```python
from build123d import *

# Parameters (mm, degrees)
BOSS_EXTRUDE1_DEPTH = 9
CUT_EXTRUDE1_DEPTH  = 1.6
CUT_EXTRUDE2_DEPTH  = 9
CUT_EXTRUDE4_DEPTH  = 6


with BuildPart() as part:
    # Sketch1 → Boss-Extrude1 (new body)
    with BuildSketch(Plane.XY):
        with BuildLine():
            Line((-290.5, 206.4), (290.5, 206.4))
            ThreePointArc((290.5, 206.4), (296.863961031, 203.763961031), (299.5, 197.4))
            Line((299.5, 197.4), (299.5, 0))
            ThreePointArc((299.5, 0), (296.863961031, -6.363961031), (290.5, -9))
            Line((290.5, -9), (-290.5, -9))
            ThreePointArc((-290.5, -9), (-296.863961031, -6.363961031), (-299.5, 0))
            Line((-299.5, 0), (-299.5, 197.4))
            ThreePointArc((-299.5, 197.4), (-296.863961031, 203.763961031), (-290.5, 206.4))
        make_face()
    extrude(amount=BOSS_EXTRUDE1_DEPTH)

    # Sketch4 → Cut-Extrude1 (cut)
    with BuildSketch(Plane.XY.offset(9)):
        with BuildLine():
            Line((-280.5, -4), (280.5, -4))
            ThreePointArc((280.5, -4), (290.399494937, 0.100505063), (294.5, 10))
            Line((294.5, 10), (294.5, 187.4))
            ThreePointArc((294.5, 187.4), (290.399494937, 197.299494937), (280.5, 201.4))
            Line((280.5, 201.4), (-280.5, 201.4))
            ThreePointArc((-280.5, 201.4), (-290.399494937, 197.299494937), (-294.5, 187.4))
            Line((-294.5, 187.4), (-294.5, 10))
            ThreePointArc((-294.5, 10), (-290.399494937, 0.100505063), (-280.5, -4))
        make_face()
        with BuildLine():
            Line((-280.5, 5), (280.5, 5))
            ThreePointArc((280.5, 5), (284.035533906, 6.464466094), (285.5, 10))
            Line((285.5, 10), (285.5, 187.4))
            ThreePointArc((285.5, 187.4), (284.035533906, 190.935533906), (280.5, 192.4))
            Line((280.5, 192.4), (-280.5, 192.4))
            ThreePointArc((-280.5, 192.4), (-284.035533906, 190.935533906), (-285.5, 187.4))
            Line((-285.5, 187.4), (-285.5, 10))
            ThreePointArc((-285.5, 10), (-284.035533906, 6.464466094), (-280.5, 5))
        make_face(mode=Mode.SUBTRACT)
    extrude(amount=-CUT_EXTRUDE1_DEPTH, mode=Mode.SUBTRACT)

    # Sketch5 → Cut-Extrude2 (cut)
    with BuildSketch(Plane.XY):
        with BuildLine():
            Line((-264.5, 177.4), (-26, 177.4))
            ThreePointArc((-26, 177.4), (-21.757359313, 175.642640687), (-20, 171.4))
            Line((-20, 171.4), (-20, 26))
            ThreePointArc((-20, 26), (-21.757359313, 21.757359313), (-26, 20))
            Line((-26, 20), (-264.5, 20))
            ThreePointArc((-264.5, 20), (-268.742640687, 21.757359313), (-270.5, 26))
            Line((-270.5, 26), (-270.5, 171.4))
            ThreePointArc((-270.5, 171.4), (-268.742640687, 175.642640687), (-264.5, 177.4))
        make_face()
        with BuildLine():
            Line((20, 171.4), (20, 26))
            ThreePointArc((20, 26), (21.757359313, 21.757359313), (26, 20))
            Line((26, 20), (163.5, 20))
            ThreePointArc((163.5, 20), (167.742640687, 21.757359313), (169.5, 26))
            Line((169.5, 26), (169.5, 171.4))
            ThreePointArc((169.5, 171.4), (167.742640687, 175.642640687), (163.5, 177.4))
            Line((163.5, 177.4), (26, 177.4))
            ThreePointArc((26, 177.4), (21.757359313, 175.642640687), (20, 171.4))
        make_face()
    extrude(amount=CUT_EXTRUDE2_DEPTH, mode=Mode.SUBTRACT)

    # Sketch7 → Cut-Extrude4 (cut)
    with BuildSketch(Plane(origin=(0, 0, 0), x_dir=(-1, 0, 0), z_dir=(0, 0, -1))):
        with BuildLine():
            Line((280.5, 26), (280.5, 171.4))
            ThreePointArc((280.5, 171.4), (275.813708499, 182.713708499), (264.5, 187.4))
            Line((264.5, 187.4), (26, 187.4))
            ThreePointArc((26, 187.4), (14.686291501, 182.713708499), (10, 171.4))
            Line((10, 171.4), (10, 26))
            ThreePointArc((10, 26), (14.686291501, 14.686291501), (26, 10))
            Line((26, 10), (264.5, 10))
            ThreePointArc((264.5, 10), (275.813708499, 14.686291501), (280.5, 26))
        make_face()
        with BuildLine():
            Line((-163.5, 10), (-26, 10))
            ThreePointArc((-26, 10), (-14.686291501, 14.686291501), (-10, 26))
            Line((-10, 26), (-10, 171.4))
            ThreePointArc((-10, 171.4), (-14.686291501, 182.713708499), (-26, 187.4))
            Line((-26, 187.4), (-163.5, 187.4))
            ThreePointArc((-163.5, 187.4), (-174.813708499, 182.713708499), (-179.5, 171.4))
            Line((-179.5, 171.4), (-179.5, 26))
            ThreePointArc((-179.5, 26), (-174.813708499, 14.686291501), (-163.5, 10))
        make_face()
    extrude(amount=-CUT_EXTRUDE4_DEPTH, mode=Mode.SUBTRACT)


solid = part.part
```
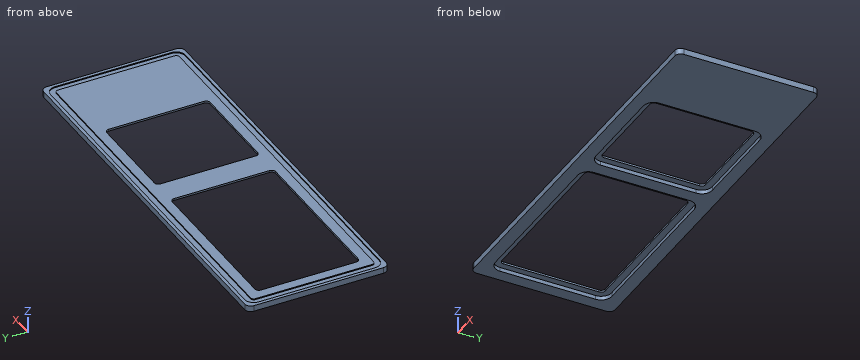
The listing builds one solid part. Answer for the finished solid, in the listing's coordinates (mm). Give positions to 0.01 mm unless a question says otherwise; leave off trailing zeros. Order: outer loops, then holes, each group sorted by start corner. A loop starts at its lowest first (then second) coordinate and runs counter-clockwise, first axis right, second up. Notation, with made-up numbers: (-14.5, 16.5) - (10.5, 16.5) arc R13 ccw to (10.5, 37.5) - close; hole circle Ø10 at (70, 42). An arc over 180 degrees is marked (long way). Answer in a Markdown table with one row per item. Add a question column.
Q1. The part is cut by section C-C (x = -210). Determine the outline of the cut face in (y, z), then the cut area to 3 significant figures.
Q2. Given P1, Ø1, axis at x = 184, y = 30.5, coming from the -Z side, flat-ended and moving along its own axis, determine where the tip first touches the part or whether it passes through.
Q3. The part is cut by section B-B (y = 133.5). Determine the outline of the cut face in (x, z), then the cut area to 3 significant figures.
Q4. Find the intervals of material crossed by line 1 along X through (y, z) = (142, 6.5); line 2 along Y through (x, z) = (77, 8); line 3 along X through (y, z) = (136, 4.5), in increasing order. Write a range as [from, to].
Q5. The part is cut by section A-A (z = 2). Determine the outline of the cut face in (x, y).
Determined:
| question | item | result |
|---|---|---|
| 1 | outline | (-9, 0) - (10, 0) - (10, 6) - (20, 6) - (20, 9) - (5, 9) - (5, 7.4) - (-4, 7.4) - (-4, 9) - (-9, 9) - close; (177.4, 6) - (187.4, 6) - (187.4, 0) - (206.4, 0) - (206.4, 9) - (201.4, 9) - (201.4, 7.4) - (192.4, 7.4) - (192.4, 9) - (177.4, 9) - close |
| 1 | area | 373 mm² |
| 2 | P1 | stops at z = 0 |
| 3 | outline | (-299.5, 0) - (-280.5, 0) - (-280.5, 6) - (-270.5, 6) - (-270.5, 9) - (-285.5, 9) - (-285.5, 7.4) - (-294.5, 7.4) - (-294.5, 9) - (-299.5, 9) - close; (-20, 6) - (-10, 6) - (-10, 0) - (10, 0) - (10, 6) - (20, 6) - (20, 9) - (-20, 9) - close; (169.5, 6) - (179.5, 6) - (179.5, 0) - (299.5, 0) - (299.5, 9) - (294.5, 9) - (294.5, 7.4) - (285.5, 7.4) - (285.5, 9) - (169.5, 9) - close |
| 3 | area | 1,520 mm² |
| 4 | line 1 | x = [-299.5, -270.5], [-20, 20], [169.5, 299.5] |
| 4 | line 2 | y = [-9, -4], [5, 20], [177.4, 192.4], [201.4, 206.4] |
| 4 | line 3 | x = [-299.5, -280.5], [-10, 10], [179.5, 299.5] |
| 5 | outline | (-299.5, 0) arc R9 ccw to (-290.5, -9) - (290.5, -9) arc R9 ccw to (299.5, 0) - (299.5, 197.4) arc R9 ccw to (290.5, 206.4) - (-290.5, 206.4) arc R9 ccw to (-299.5, 197.4) - close; hole (-280.5, 26) arc R16 ccw to (-264.5, 10) - (-26, 10) arc R16 ccw to (-10, 26) - (-10, 171.4) arc R16 ccw to (-26, 187.4) - (-264.5, 187.4) arc R16 ccw to (-280.5, 171.4) - close; hole (10, 26) arc R16 ccw to (26, 10) - (163.5, 10) arc R16 ccw to (179.5, 26) - (179.5, 171.4) arc R16 ccw to (163.5, 187.4) - (26, 187.4) arc R16 ccw to (10, 171.4) - close |
